from build123d import *

# Parameters (mm, degrees)
ESQUISSE1_R             = 3.15
ESQUISSE1_R_2           = 1.15
ESQUISSE1_W             = 13.4
ESQUISSE1_H             = 12.4
BOSS_EXTRU_1_DEPTH      = 3
ESQUISSE2_W             = 14
ESQUISSE2_H             = 13
ENL_V_MAT_EXTRU_1_DEPTH = 2
CONG_1_R                = 12
ESQUISSE3_W             = 25
ESQUISSE3_H             = 2
ENL_V_MAT_EXTRU_2_DEPTH = 19.153374342
CONG_2_DEPTH            = 4
BOSS_EXTRU_3_DEPTH      = 3
CONG_4_R                = 0.5
CONG_5_R                = 0.2
SYM_TRIE2_START         = 3
SYM_TRIE2_DEPTH         = 3


with BuildPart() as part:
    # Esquisse1 → Boss.-Extru.1 (new body)
    # profile 1 of 6: a face of its own
    with BuildSketch(Plane.XY):
        with Locations((-9, 10)):
            Circle(ESQUISSE1_R)
        with Locations((-9, 10)):
            Circle(ESQUISSE1_R_2, mode=Mode.SUBTRACT)
    # profile 2 of 6: a face of its own
    with BuildSketch(Plane.XY):
        with BuildLine():
            ThreePointArc((-5.85, 10), (-6.66895946, 7.881332966), (-8.7, 6.864318256))
            Line((-8.7, 6.864318256), (-8.7, -6.864318256))
            ThreePointArc((-8.7, -6.864318256), (-6.66895946, -7.881332966), (-5.85, -10))
            ThreePointArc((-5.85, -10), (-5.909952225, -10.611641029), (-6.087526824, -11.2))
            Line((-6.087526824, -11.2), (6.087526824, -11.2))
            ThreePointArc((6.087526824, -11.2), (6.301939581, -8.374278629), (8.7, -6.864318256))
            Line((8.7, -6.864318256), (8.7, 6.864318256))
            ThreePointArc((8.7, 6.864318256), (6.301939581, 8.374278629), (6.087526824, 11.2))
            Line((6.087526824, 11.2), (-6.087526824, 11.2))
            ThreePointArc((-6.087526824, 11.2), (-5.909952225, 10.611641029), (-5.85, 10))
        make_face()
        Rectangle(ESQUISSE1_W, ESQUISSE1_H, mode=Mode.SUBTRACT)
    # profile 3 of 6: a face of its own
    with BuildSketch(Plane.XY):
        with Locations((9, 10)):
            Circle(ESQUISSE1_R)
        with Locations((9, 10)):
            Circle(ESQUISSE1_R_2, mode=Mode.SUBTRACT)
    # profile 4 of 6: a face of its own
    with BuildSketch(Plane.XY):
        with Locations((9, -10)):
            Circle(ESQUISSE1_R)
        with Locations((9, -10)):
            Circle(ESQUISSE1_R_2, mode=Mode.SUBTRACT)
    # profile 5 of 6: a face of its own
    with BuildSketch(Plane.XY):
        with Locations((-9, -10)):
            Circle(ESQUISSE1_R)
        with Locations((-9, -10)):
            Circle(ESQUISSE1_R_2, mode=Mode.SUBTRACT)
    # profile 6 of 6: a face of its own
    with BuildSketch(Plane.XY):
        Rectangle(ESQUISSE1_W, ESQUISSE1_H)
    extrude(amount=BOSS_EXTRU_1_DEPTH)

    # Esquisse2 → Enlèv. mat.-Extru.1 (cut)
    with BuildSketch(Plane(origin=(0, 0, 0), x_dir=(-1, 0, 0), z_dir=(0, 0, -1))):
        Rectangle(ESQUISSE2_W, ESQUISSE2_H)
    extrude(amount=-ENL_V_MAT_EXTRU_1_DEPTH, mode=Mode.SUBTRACT)

    # Congé1
    cong_1_edges = [part.edges().sort_by_distance(p)[0] for p in [
        (8.7, 6.864318256, 1.5),
        (8.7, -6.864318256, 1.5),
        (-8.7, -6.864318256, 1.5),
        (-8.7, 6.864318256, 1.5),
    ]]
    fillet(cong_1_edges, radius=CONG_1_R)

    # Esquisse3 → Enlèv. mat.-Extru.2 (cut, through all)
    with BuildSketch(Plane.XY.offset(3)):
        with Locations((0, -13.5)):
            Rectangle(ESQUISSE3_W, ESQUISSE3_H)
        with Locations((0, 13.5)):
            Rectangle(ESQUISSE3_W, ESQUISSE3_H)
    extrude(amount=-ENL_V_MAT_EXTRU_2_DEPTH, mode=Mode.SUBTRACT)

    # Congé2: read off the stored shape, not the designer's step
    # Congé2 outline → Congé2 (cut)
    with BuildSketch(Plane.XY):
        with BuildLine():
            ThreePointArc((-11.432673267, 7.998850137), (-11.302722907, 7.838074648), (-11.175561441, 7.675084417))
            ThreePointArc((-11.175561441, 7.675084417), (-11.484688477, 10.827639494), (-8.794451801, 12.5))
            Line((-8.794451801, 12.5), (-10.91637679, 12.5))
            ThreePointArc((-10.91637679, 12.5), (-12.129480248, 10.358961527), (-11.432673267, 7.998850137))
        make_face()
        with BuildLine():
            Line((-7.08362321, 12.5), (-8.559368243, 12.5))
            ThreePointArc((-8.559368243, 12.5), (-7.162944239, 12.155183609), (-6.087526824, 11.2))
            ThreePointArc((-6.087526824, 11.2), (-6.499610431, 11.915868472), (-7.08362321, 12.5))
        make_face()
        with BuildLine():
            Line((10.91637679, 12.5), (8.794451801, 12.5))
            ThreePointArc((8.794451801, 12.5), (11.484688477, 10.827639494), (11.175561441, 7.675084417))
            ThreePointArc((11.175561441, 7.675084417), (11.302722907, 7.838074648), (11.432673267, 7.998850137))
            ThreePointArc((11.432673267, 7.998850137), (12.129480248, 10.358961527), (10.91637679, 12.5))
        make_face()
        with BuildLine():
            ThreePointArc((6.087526824, 11.2), (7.162944239, 12.155183609), (8.559368243, 12.5))
            Line((8.559368243, 12.5), (7.08362321, 12.5))
            ThreePointArc((7.08362321, 12.5), (6.499610431, 11.915868472), (6.087526824, 11.2))
        make_face()
        with BuildLine():
            ThreePointArc((11.432673267, -7.998850137), (11.302722907, -7.838074648), (11.175561441, -7.675084417))
            ThreePointArc((11.175561441, -7.675084417), (11.484688477, -10.827639494), (8.794451801, -12.5))
            Line((8.794451801, -12.5), (10.91637679, -12.5))
            ThreePointArc((10.91637679, -12.5), (12.129480248, -10.358961527), (11.432673267, -7.998850137))
        make_face()
        with BuildLine():
            Line((7.08362321, -12.5), (8.559368243, -12.5))
            ThreePointArc((8.559368243, -12.5), (7.162944239, -12.155183609), (6.087526824, -11.2))
            ThreePointArc((6.087526824, -11.2), (6.499610431, -11.915868472), (7.08362321, -12.5))
        make_face()
        with BuildLine():
            ThreePointArc((-7.08362321, -12.5), (-6.499610431, -11.915868472), (-6.087526824, -11.2))
            ThreePointArc((-6.087526824, -11.2), (-7.162944239, -12.155183609), (-8.559368243, -12.5))
            Line((-8.559368243, -12.5), (-7.08362321, -12.5))
        make_face()
        with BuildLine():
            Line((-10.91637679, -12.5), (-8.794451801, -12.5))
            ThreePointArc((-8.794451801, -12.5), (-11.484688477, -10.827639494), (-11.175561441, -7.675084417))
            ThreePointArc((-11.175561441, -7.675084417), (-11.302722907, -7.838074648), (-11.432673267, -7.998850137))
            ThreePointArc((-11.432673267, -7.998850137), (-12.129480248, -10.358961527), (-10.91637679, -12.5))
        make_face()
    extrude(amount=CONG_2_DEPTH, mode=Mode.SUBTRACT)

    # Esquisse5 → Boss.-Extru.3 (add)
    with BuildSketch(Plane.XY.offset(3)):
        with BuildLine():
            Line((-10.253049234, 8), (-9.010874707, 8))
            ThreePointArc((-9.010874707, 8), (-6.5, 0), (-9.010874707, -8))
            Line((-9.010874707, -8), (-10.253049234, -8))
            ThreePointArc((-10.253049234, -8), (-7.5, 0), (-10.253049234, 8))
        make_face()
        with BuildLine():
            Line((-8.375702269, -8.5), (-7.140792906, -8.5))
            ThreePointArc((-7.140792906, -8.5), (-4.5, 0), (-7.140792906, 8.5))
            Line((-7.140792906, 8.5), (-8.375702269, 8.5))
            ThreePointArc((-8.375702269, 8.5), (-5.5, 0), (-8.375702269, -8.5))
        make_face()
        with BuildLine():
            Line((-6.5, 9), (-5.271243445, 9))
            ThreePointArc((-5.271243445, 9), (-2.5, 0), (-5.271243445, -9))
            Line((-5.271243445, -9), (-6.5, -9))
            ThreePointArc((-6.5, -9), (-3.5, 0), (-6.5, 9))
        make_face()
        with BuildLine():
            Line((-4.62560681, 9.5), (-3.40212782, 9.5))
            ThreePointArc((-3.40212782, 9.5), (-0.5, 0), (-3.40212782, -9.5))
            Line((-3.40212782, -9.5), (-4.62560681, -9.5))
            ThreePointArc((-4.62560681, -9.5), (-1.5, 0), (-4.62560681, 9.5))
        make_face()
        with BuildLine():
            Line((-2.752272915, 10), (-1.533370453, 10))
            ThreePointArc((-1.533370453, 10), (-0.704242426, 8.630993145), (0, 7.193747285))
            ThreePointArc((0, 7.193747285), (0.704242426, 8.630993145), (1.533370453, 10))
            Line((1.533370453, 10), (2.752272915, 10))
            ThreePointArc((2.752272915, 10), (1.090413162, 7.179459136), (0, 4.092676386))
            ThreePointArc((0, 4.092676386), (-1.090413162, 7.179459136), (-2.752272915, 10))
        make_face()
        with BuildLine():
            Line((-2.752272915, -10), (-1.533370453, -10))
            ThreePointArc((-1.533370453, -10), (-0.704242426, -8.630993145), (0, -7.193747285))
            ThreePointArc((0, -7.193747285), (0.704242426, -8.630993145), (1.533370453, -10))
            Line((1.533370453, -10), (2.752272915, -10))
            ThreePointArc((2.752272915, -10), (1.090413162, -7.179459136), (0, -4.092676386))
            ThreePointArc((0, -4.092676386), (-1.090413162, -7.179459136), (-2.752272915, -10))
        make_face()
    extrude(amount=BOSS_EXTRU_3_DEPTH)

    # Congé4
    cong_4_edges = [part.edges().sort_by_distance(p)[0] for p in [
        (2.752272915, 10, 4.5),
        (1.533370453, 10, 4.5),
        (0, 7.193747285, 4.5),
        (-1.533370453, 10, 4.5),
        (-2.752272915, 10, 4.5),
        (-3.40212782, 9.5, 4.5),
        (-4.62560681, 9.5, 4.5),
        (-5.271243445, 9, 4.5),
        (-6.5, 9, 4.5),
        (-7.140792906, 8.5, 4.5),
        (-8.375702269, 8.5, 4.5),
        (-9.010874707, 8, 4.5),
        (-10.253049234, 8, 4.5),
        (0, -7.193747285, 4.5),
        (2.752272915, -10, 4.5),
        (1.533370453, -10, 4.5),
        (-1.533370453, -10, 4.5),
        (-2.752272915, -10, 4.5),
        (-3.40212782, -9.5, 4.5),
        (-4.62560681, -9.5, 4.5),
        (-5.271243445, -9, 4.5),
        (-6.5, -9, 4.5),
        (-7.140792906, -8.5, 4.5),
        (-8.375702269, -8.5, 4.5),
        (-9.010874707, -8, 4.5),
        (-10.253049234, -8, 4.5),
    ]]
    fillet(cong_4_edges, radius=CONG_4_R - 0.0001)  # a hair under: the kernel refuses the full size

    # Congé5
    cong_5_edges = [part.edges().sort_by_distance(p)[0] for p in [
        (0, 4.092676386, 4.5),
        (0, -4.092676386, 4.5),
    ]]
    fillet(cong_5_edges, radius=CONG_5_R)

    # Symétrie2: read off the stored shape, not the designer's step
    # Symétrie2 outline → Symétrie2 (add)
    with BuildSketch(Plane.XY.offset(SYM_TRIE2_START)):
        with BuildLine():
            ThreePointArc((9.27502784, -8), (9.715986392, -7.73570226), (9.690767549, -7.222222222))
            ThreePointArc((9.690767549, -7.222222222), (7.5, 0), (9.690767549, 7.222222222))
            ThreePointArc((9.690767549, 7.222222222), (9.715986392, 7.73570226), (9.27502784, 8))
            ThreePointArc((9.27502784, 8), (9.039325579, 7.940958552), (8.85928813, 7.777777778))
            ThreePointArc((8.85928813, 7.777777778), (6.5, 0), (8.85928813, -7.777777778))
            ThreePointArc((8.85928813, -7.777777778), (9.039325579, -7.940958552), (9.27502784, -8))
        make_face()
        with BuildLine():
            ThreePointArc((7.406613378, -8.5), (7.847028542, -8.236716038), (7.823626709, -7.724137931))
            ThreePointArc((7.823626709, -7.724137931), (5.5, 0), (7.823626709, 7.724137931))
            ThreePointArc((7.823626709, 7.724137931), (7.847028542, 8.236716038), (7.406613378, 8.5))
            ThreePointArc((7.406613378, 8.5), (7.169897339, 8.440415165), (6.989600046, 8.275862069))
            ThreePointArc((6.989600046, 8.275862069), (4.5, 0), (6.989600046, -8.275862069))
            ThreePointArc((6.989600046, -8.275862069), (7.169897339, -8.440415165), (7.406613378, -8.5))
        make_face()
        with BuildLine():
            ThreePointArc((5.538518603, -9), (5.978459948, -8.737595482), (5.956630906, -8.225806452))
            ThreePointArc((5.956630906, -8.225806452), (3.5, 0), (5.956630906, 8.225806452))
            ThreePointArc((5.956630906, 8.225806452), (5.978459948, 8.737595482), (5.538518603, 9))
            ThreePointArc((5.538518603, 9), (5.300923121, 8.939941345), (5.1204063, 8.774193548))
            ThreePointArc((5.1204063, 8.774193548), (2.5, 0), (5.1204063, -8.774193548))
            ThreePointArc((5.1204063, -8.774193548), (5.300923121, -8.939941345), (5.538518603, -9))
        make_face()
        with BuildLine():
            ThreePointArc((3.670683314, -9.5), (4.110207851, -9.238365647), (4.089753517, -8.727272727))
            ThreePointArc((4.089753517, -8.727272727), (1.5, 0), (4.089753517, 8.727272727))
            ThreePointArc((4.089753517, 8.727272727), (4.110207851, 9.238365647), (3.670683314, 9.5))
            ThreePointArc((3.670683314, 9.5), (3.432317667, 9.439524536), (3.251613111, 9.272727273))
            ThreePointArc((3.251613111, 9.272727273), (0.5, 0), (3.251613111, -9.272727273))
            ThreePointArc((3.251613111, -9.272727273), (3.432317667, -9.439524536), (3.670683314, -9.5))
        make_face()
    extrude(amount=SYM_TRIE2_DEPTH)


solid = part.part
Design review of the part built by this model. Coordinates are the model's own, in mm. A direction names the side the tool comes from. Coordinates: 2 decimals unless noted, no trailing zeros. Order: outer loops, then holes, each group sorted by start corner. A loop starts at its lowest first (then second) coordinate and runs counter-clockwise, first axis right, second up. Notation, with made-up numbers: (7, -37) - (55, -37) arc R22 cw to (55, -26) - close; hole circle Ø2 at (14.25, 14). An arc over 180 degrees is marked (long way). Put each result on its own line as item: value.
1) The part is to be moulded in two halves that separate along Y. For faces 1 (the face through (7, 1, 6)), 2 (the face through (11.464, 10.869, 1.479)), 3 (the face through (0, 11.2, 1)), say which applies: released by +Y, released by -Y, zero draft, split by the parting line, or undercut.
Response values:
face 1: zero draft
face 2: undercut
face 3: released by +Y
2) Wall thickness on L1, parallel to Y at x = -3, z = 1; L2, parallel to Y at x = 8.25, z = 0.75; L3, parallel to X at y = -9.25, z = 0.5: over which ranges is each line inside the solid? List them lowest first. Write a range as from..to.
Response values:
L1: y = -11.2..-6.5, 6.5..11.2
L2: y = -12.48..-10.87, -9.13..9.13, 10.87..12.48
L3: x = -11.78..-9.87, -8.13..8.13, 9.87..11.78
3) Take a section at B-B, the plane z = 3.5. Count the separate pieces of the cut face and the enclosed holes in it, and give its area (3 significant figures).
Response values:
separate pieces: 10
enclosed holes: 0
area: 165 mm²
4) Tool access review of faces 4 (the face through (7.181, -12.165, 1.479)), 5 (the face through (1.062, 7.119, 4.479)), 6 (the face through (-7.181, 12.165, 1.479)), 7 (the face through (-0.9, 8.98, 4.48)), 8 (the face through (-7, 1, 6)): name each direction out of +Z, -Z, +X, -X, +Y, -Y from which nothing blocks a thin tool from reaching the whole face with its end or side.
Response values:
face 4: +Z, -Z, -Y
face 5: +Z
face 6: +Z, -Z, +Y
face 7: +Z, +Y
face 8: +Z, +X, -X, +Y, -Y
5) Take a section at A-A, the plane z = 0.5. Give the boundary of the cut face in (x, y), and give its area (3 significant figures).
Response values:
outline: (-11.18, -7.68) arc R3 ccw to (-8.79, -12.5) - (-8.56, -12.5) arc R3 ccw to (-6.09, -11.2) - (6.09, -11.2) arc R3 ccw to (8.56, -12.5) - (8.79, -12.5) arc R3 ccw to (11.18, -7.68) arc R12 cw to (8.7, -0.38) - (8.7, 0.38) arc R12 cw to (11.18, 7.68) arc R3 ccw to (8.79, 12.5) - (8.56, 12.5) arc R3 ccw to (6.09, 11.2) - (-6.09, 11.2) arc R3 ccw to (-8.56, 12.5) - (-8.79, 12.5) arc R3 ccw to (-11.18, 7.68) arc R12 cw to (-8.7, 0.38) - (-8.7, -0.38) arc R12 cw to start; hole circle Ø2.3 at (-9, -10); hole circle Ø2.3 at (-9, 10); hole (-7, -6.5) - (7, -6.5) - (7, 6.5) - (-7, 6.5) - close; hole circle Ø2.3 at (9, -10); hole circle Ø2.3 at (9, 10)
area: 274 mm²
6) Insertion check: P1, Ø3.5, axis at x = 2, z = 1.5, coming from the +Y side; P2, Ø1, axis at x = -3.5, z = 1, coming from the -Y side; P3, Ø8, axis at x = 7.5, y = 8.5, coming from the -Z side; P4, Ø3, axis at y = 0, z = 3.5, coming from the +X side. Each pin has a flat end and moves straight along its axis. Give the tip position at first contact, or say it passes through.
Response values:
P1: stops at y = 11.2
P2: stops at y = -11.2
P3: stops at z = 0
P4: stops at x = 8.75
